For this review, take the finished solid that the model builds, in its own axes (mm). A direction names the side the tool comes from. Coordinates: 2 decimals unless noted, no trailing zeros. Write each loop counter-clockwise with the first axis right and the second up, starting at its lowest first coordinate (ties: lowest second). Pieces come first, ordered by that corner, then holes. Notation, with made-up numbers: M -19.5,62.5 L 30.5,62.5 A23 ccw 30.5,75.5 Z; hole C 9.5,-18 d4. An arc over 180 degrees is marked long. One line per question, with ' | ' between items.
from build123d import *

# Parameters (mm, degrees)
ESBO_O1_R                = 12.5
RESSALTO_EXTRUS_O1_DEPTH = 1
ESBO_O2_R                = 11.5
RESSALTO_EXTRUS_O2_DEPTH = 15
ESBO_O3_R                = 12.5
RESSALTO_EXTRUS_O3_DEPTH = 1
CORTE_EXTRUS_O1_DEPTH    = 12
CORTE_EXTRUS_O2_DEPTH    = 35
CORTE_EXTRUS_O3_START    = -5
ESBO_O7_R                = 2.75
CORTE_EXTRUS_O3_DEPTH    = 35
ESBO_O8_R                = 9.5
CORTE_EXTRUS_O4_DEPTH    = 11
ESBO_O9_W                = 5.8
ESBO_O9_H                = 2.5
CORTE_EXTRUS_O5_DEPTH    = 4.8


with BuildPart() as part:
    # Esboço1 → Ressalto-extrusão1 (new body)
    with BuildSketch(Plane(origin=(0, 0, 0), x_dir=(1, 0, 0), z_dir=(0, 1, 0))):
        with Locations(Location((0, 0, 0), (0, 0, 270))):
            Circle(ESBO_O1_R)
    extrude(amount=RESSALTO_EXTRUS_O1_DEPTH)

    # Esboço2 → Ressalto-extrusão2 (add)
    with BuildSketch(Plane(origin=(0, 1, 0), x_dir=(1, 0, 0), z_dir=(0, 1, 0))):
        with Locations(Location((0, 0, 0), (0, 0, 270))):
            Circle(ESBO_O2_R)
    extrude(amount=RESSALTO_EXTRUS_O2_DEPTH)

    # Esboço3 → Ressalto-extrusão3 (add)
    with BuildSketch(Plane(origin=(0, 16, 0), x_dir=(1, 0, 0), z_dir=(0, 1, 0))):
        with Locations(Location((0, 0, 0), (0, 0, 270))):
            Circle(ESBO_O3_R)
    extrude(amount=RESSALTO_EXTRUS_O3_DEPTH)

    # Esboço4 → Corte-extrusão1 (cut)
    with BuildSketch(Plane(origin=(0, 17, 0), x_dir=(1, 0, 0), z_dir=(0, 1, 0))):
        with BuildLine():
            ThreePointArc((-1.44222051, 0.9), (-1.486606875, -0.824621125), (0, -1.7))
            Line((0, -1.7), (0, 0.9))
            Line((0, 0.9), (-1.44222051, 0.9))
        make_face()
        with BuildLine():
            Line((0, 0.9), (0, -1.7))
            ThreePointArc((0, -1.7), (1.202081528, -1.202081528), (1.7, 0))
            ThreePointArc((1.7, 0), (1.634284992, 0.468094613), (1.44222051, 0.9))
            Line((1.44222051, 0.9), (0, 0.9))
        make_face()
    extrude(amount=-CORTE_EXTRUS_O1_DEPTH, mode=Mode.SUBTRACT)

    # Esboço6 → Corte-extrusão2 (cut)
    with BuildSketch(Plane.XY):
        with BuildLine():
            ThreePointArc((0, 14.5), (-1.5, 13), (0, 11.5))
            Line((0, 11.5), (0, 13))
            Line((0, 13), (0, 14.5))
        make_face()
        with BuildLine():
            Line((0, 13), (0, 11.5))
            ThreePointArc((0, 11.5), (1.060660172, 11.939339828), (1.5, 13))
            ThreePointArc((1.5, 13), (1.060660172, 14.060660172), (0, 14.5))
            Line((0, 14.5), (0, 13))
        make_face()
    extrude(amount=-CORTE_EXTRUS_O2_DEPTH, mode=Mode.SUBTRACT)

    # Esboço7 → Corte-extrusão3 (cut)
    with BuildSketch(Plane.XY.offset(CORTE_EXTRUS_O3_START)):
        with Locations((0, 13)):
            Circle(ESBO_O7_R)
    extrude(amount=-CORTE_EXTRUS_O3_DEPTH, mode=Mode.SUBTRACT)

    # Esboço8 → Corte-extrusão4 (cut)
    with BuildSketch(Plane(origin=(0, 0, 0), x_dir=(-1, 0, 0), z_dir=(0, -1, 0))):
        with Locations(Location((0, 0, 0), (0, 0, 90))):
            Circle(ESBO_O8_R)
    extrude(amount=-CORTE_EXTRUS_O4_DEPTH, mode=Mode.SUBTRACT)

    # Esboço9 → Corte-extrusão5 (cut)
    with BuildSketch(Plane.XZ.offset(-11)):
        with Locations((0, -2.700284177)):
            Rectangle(ESBO_O9_W, ESBO_O9_H)
    extrude(amount=-CORTE_EXTRUS_O5_DEPTH, mode=Mode.SUBTRACT)


solid = part.part
1. Take a section at B-B on z = 2.75. State the section outline as (x, y) points.
Computed values:
outline: M -12.19,0 L -9.09,0 L -9.09,11 L 9.09,11 L 9.09,0 L 12.19,0 L 12.19,1 L 11.17,1 L 11.17,16 L 12.19,16 L 12.19,17 L -12.19,17 L -12.19,16 L -11.17,16 L -11.17,1 L -12.19,1 Z
2. Draft analysis for pull direction Z (two halves, no side actions). For faces 1 (the flat face through (0, 15.8, -3)), 2 (the cylindrical face through (3.755, 16.493, 11.923)), 3 (the flat face through (-11, 16, 4)), state which applies: pulls with the +Z half, pulls with the -Z half, needs draft (parallel to the pull), parting line crosses it, or undercut.
Computed values:
face 1: undercut | face 2: parting line crosses it | face 3: needs draft
3. Clearance check with flat-ended pins moving along their axes: P1, Ø3, axis at y = 13, z = -2.5, coming from the +X side; P2, Ø4.5, axis at x = 0, y = 13, coming from the -Z side; P3, Ø1.5, axis at y = 4, z = 3.5, coming from the -X side; P4, Ø8, axis at x = 2, z = 6.5, coming from the -Y side. State where each tip first meets the part, or that it passes through.
Computed values:
P1: stops at x = 11.46 | P2: stops at z = -5 | P3: stops at x = -11.17 | P4: stops at y = 0
4. Take a section at A-A on y = 1.75. State the section outline as (x, z) points.
Computed values:
outline: C 0,0 d23; hole C 0,0 d19
5. For line 1 along Z through (x, y) = (0, 5.25); line 2 along Y through (x, z) = (-5.75, 4.5); line 3 along X through (y, z) = (13, -6.75), list the stretches that pass through material, from the lowest coordinate up.
Computed values:
line 1: z = -11.5 to -9.5, 9.5 to 11.5 | line 2: y = 11 to 17 | line 3: x = -9.31 to -2.75, 2.75 to 9.31
6. Take a section at D-D on z = -6.75. State the section outline as (x, y) points, plus the area to 3 significant figures.
Computed values:
outline: M -10.52,0 L -6.68,0 L -6.68,11 L -1.89,11 A2.75 cw long 1.89,11 L 6.68,11 L 6.68,0 L 10.52,0 L 10.52,1 L 9.31,1 L 9.31,16 L 10.52,16 L 10.52,17 L -10.52,17 L -10.52,16 L -9.31,16 L -9.31,1 L -10.52,1 Z | area: 153 mm2
7. Take a section at C-C on x = -5.75. State the section outline as (y, z) points, plus the area to 3 significant figures.
Computed values:
outline: M 0,-11.1 L 1,-11.1 L 1,-9.96 L 16,-9.96 L 16,-11.1 L 17,-11.1 L 17,11.1 L 16,11.1 L 16,9.96 L 1,9.96 L 1,11.1 L 0,11.1 L 0,7.56 L 11,7.56 L 11,-7.56 L 0,-7.56 Z | area: 177 mm2
8. Machinability: for faces 4 (the flat face through (0, 11.3, -0.9)), 5 (the flat face through (-2, 11, 0)), 6 (the flat face through (0, 15, -5)), 7 (the flat face through (-11, 1, 4)), which of the approach directions +Z, -Z, +X, -X, +Y, -Y give a long, thin tool a straight path to every point of the face, cutting with its end or side? Answer none if there is none.
Computed values:
face 4: +Y, -Y | face 5: -Y | face 6: -Z | face 7: none
